from build123d import *

# Parameters (mm, degrees)
SKETCH_1_W          = 26
SKETCH_1_H          = 30
EXTRUDE_1_DEPTH     = 5
SKETCH_2_R          = 1.85
CUT_EXTRUDE_1_DEPTH = 12
EXTRUDE_START       = 8
EXTRUDE_2_DEPTH     = 8
SKETCH_5_R          = 1.85
CUT_EXTRUDE_2_DEPTH = 33.015621187
SKETCH_6_R          = 1.15
CUT_EXTRUDE_3_DEPTH = 8


with BuildPart() as part:
    # 草图1 → 凸台-拉伸1 (new body)
    with BuildSketch(Plane.XY):
        with Locations((13, -15)):
            Rectangle(SKETCH_1_W, SKETCH_1_H)
    extrude(amount=EXTRUDE_1_DEPTH)

    # 草图2 → 切除-拉伸1 (cut)
    with BuildSketch(Plane(origin=(0, 0, 0), x_dir=(1, 0, 0), z_dir=(0, 1, 0))):
        with Locations((3, -5)):
            Circle(SKETCH_2_R)
        with Locations((23, -5)):
            Circle(SKETCH_2_R)
    extrude(amount=-CUT_EXTRUDE_1_DEPTH, mode=Mode.SUBTRACT)

    # 草图4 → 凸台-拉伸2 (add)
    with BuildSketch(Plane(origin=(0, -12, 0), x_dir=(1, 0, 0), z_dir=(0, 1, 0)).offset(EXTRUDE_START)):
        with BuildLine():
            Line((1.412549213, -4.05), (4.587450787, -4.05))
            ThreePointArc((4.587450787, -4.05), (3, -3.15), (1.412549213, -4.05))
        make_face()
        with BuildLine():
            Line((21.412549213, -4.05), (24.587450787, -4.05))
            ThreePointArc((24.587450787, -4.05), (23, -3.15), (21.412549213, -4.05))
        make_face()
    extrude(amount=-EXTRUDE_2_DEPTH)

    # 草图5 → 切除-拉伸2 (cut, through all)
    with BuildSketch(Plane(origin=(0, -12, 0), x_dir=(1, 0, 0), z_dir=(0, 1, 0))):
        with Locations((3, -5)):
            Circle(SKETCH_5_R)
        with Locations((23, -5)):
            Circle(SKETCH_5_R)
    extrude(amount=-CUT_EXTRUDE_2_DEPTH, mode=Mode.SUBTRACT)

    # 草图6 → 切除-拉伸3 (cut)
    with BuildSketch(Plane(origin=(0, 0, 0), x_dir=(-1, 0, 0), z_dir=(0, 0, -1))):
        with Locations((-18, -15)):
            Circle(SKETCH_6_R)
        with Locations((-8, -15)):
            Circle(SKETCH_6_R)
    extrude(amount=-CUT_EXTRUDE_3_DEPTH, mode=Mode.SUBTRACT)


solid = part.part
Geometry: final body of the model. Coordinates: model frame, mm. A direction names the side the tool comes from. Give positions to 0.01 mm unless a question says otherwise; leave off trailing zeros. Order: outer loops, then holes, each group sorted by start corner. A loop starts at its lowest first (then second) coordinate and runs counter-clockwise, first axis right, second up. Notation, with made-up numbers: (21, 32.5) -> (39, 32.5) arc R32 ccw to (39, 60.5) -> close; hole circle Ø7 at (-20, 6). An arc over 180 degrees is marked (long way). Answer as a JSON object with one key per item and string values.
Q1. First-contact query: pin 1 (0.7 mm diameter, centred on x = 3, z = 4, fed in from -Y); pin 2 (1 mm diameter, centred on x = 2.5, y = -8.5, fed in from +Z); pin 3 (1.8 mm diameter, centred on x = 18, y = -15, fed in from +Z); pin 4 (0.5 mm diameter, centred on x = 23, z = 3.5, fed in from +Y). Flat tips, straight axial feed; report the tip coordinate or a pass-through.
Entries:
{"pin 1": "stops at y = -12", "pin 2": "stops at z = 4.05", "pin 3": "passes through", "pin 4": "stops at y = -4"}
Q2. Section C-C (x = 23). Output: boundary loops of the cut face in (y, z), plus the area to 3 significant figures.
Entries:
{"outline": "(-30, 0) -> (0, 0) -> (0, 3.15) -> (-4, 3.15) -> (-4, 4.05) -> (-12, 4.05) -> (-12, 3.15) -> (-30, 3.15) -> close", "area": "102 mm^2"}
Q3. Section A-A (x = 18). Output: boundary loops of the cut face in (y, z).
Entries:
{"outline": "(-30, 0) -> (-16.15, 0) -> (-16.15, 5) -> (-30, 5) -> close; (-13.85, 0) -> (0, 0) -> (0, 5) -> (-13.85, 5) -> close"}
Q4. Draft query along X for faces 5 (the cylindrical face through (3.04, -18.12, 3.15)), 6 (the flat face through (13, 0, 2)), 7 (the flat face through (26, -15, 2)). Return one class per face: released by +X, released by -X, zero draft, split by the parting line, or undercut.
Entries:
{"face 5": "undercut", "face 6": "zero draft", "face 7": "released by +X"}
Q5. Access query for faces 1 (the flat face through (23, -12, 3.7)), 2 (the flat face through (3, -4, 3.7)), 3 (the flat face through (13, -15, 0)), 4 (the flat face through (23, -8, 4.05)). Directions: +Z, -Z, +X, -X, +Y, -Y. A direction counts if a zero-diameter tool reaches every point of the face in a straight line with its end or side. Return the directions, or none.
Entries:
{"face 1": "+Z, -Y", "face 2": "+Z, +Y", "face 3": "-Z, +X, -X, +Y, -Y", "face 4": "+Z, +Y, -Y"}
Q6. Section B-B (y = -7.25). Output: boundary loops of the cut face in (x, z).
Entries:
{"outline": "(0, 0) -> (26, 0) -> (26, 5) -> (24.85, 5) arc R1.85 cw to (24.59, 4.05) -> (21.41, 4.05) arc R1.85 cw to (21.15, 5) -> (4.85, 5) arc R1.85 cw to (4.59, 4.05) -> (1.41, 4.05) arc R1.85 cw to (1.15, 5) -> (0, 5) -> close"}
Q7. Material intervals for probe 1 along Y at (x, z) = (8, 2.75); probe 2 along X at (y, z) = (-24.25, 4.25); probe 3 along Z at (x, y) = (23, -7), sorted ascending.
Entries:
{"probe 1": "y = -30 to -16.15, -13.85 to 0", "probe 2": "x = 0 to 1.31, 4.69 to 21.31, 24.69 to 26", "probe 3": "z = 0 to 4.05"}
Q8. Section D-D (y = -27). Output: boundary loops of the cut face in (x, z), plus the area to 3 significant figures.
Entries:
{"outline": "(0, 0) -> (26, 0) -> (26, 5) -> (24.85, 5) arc R1.85 cw to (21.15, 5) -> (4.85, 5) arc R1.85 cw to (1.15, 5) -> (0, 5) -> close", "area": "119 mm^2"}
